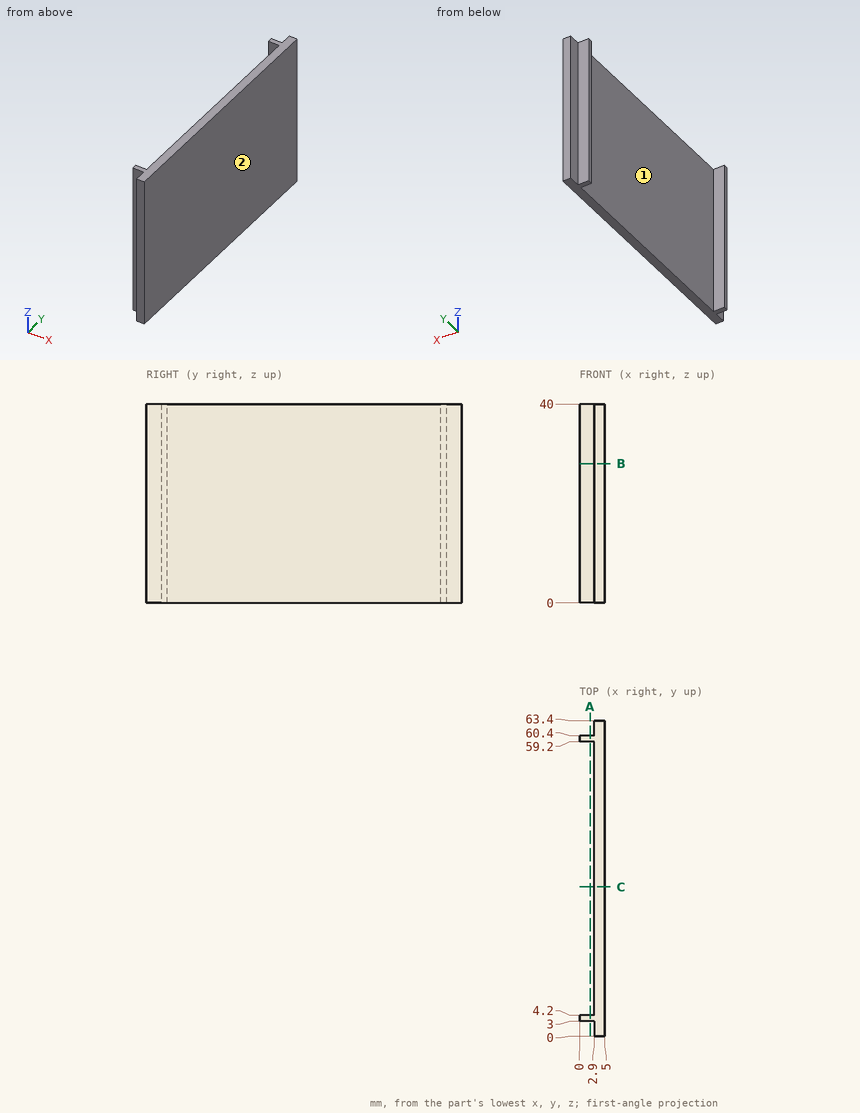
For this review, use the dimensioned drawing (mm, ordinates from the lowest corner) and the shaded views. Coordinates: 2 decimals unless noted, no trailing zeros. Loops run counter-clockwise (first coordinate to the right, second up) from the corner with the lowest first, then second, coordinate; pieces in that order, holes last. Notation, with made-up numbers: (44, 34.5) - (99, 34.5) arc R17 cw to (99, 57.5) - close; hole circle Ø6 at (81.5, 77). An arc over 180 degrees is marked (long way). Use one line per item in the form item = value. Start each with the question number.
1) Draft analysis for pull direction Y (two halves, no side actions). For the marked faces 1 and 2, state which applies: released by +Y, released by -Y, zero draft, split by the parting line, or undercut.
2) For pin 1 (0.9 mm diameter, centred on y = 62, z = 24.5, fed in from -X); pin 2 (3 mm diameter, centred on x = 2, z = 17, fed in from -Y); pin 3 (0.9 mm diameter, centred on x = 1.5, z = 20, fed in from -Y); pin 4 (1.4 mm diameter, centred on x = 2, z = 29, fed in from +Y), all flat-tipped, find the tip position at first contact; note any pin that passes through.
3) To check wall thickness, follow probe 1 along Y at (x, z) = (1.15, 11); probe 2 along X at (y, z) = (59, 29). State the ranges of each line that lie inside material, in increasing order. Write a range as from..to.
4) Take a section at A-A (x = 2.1). State the section outline as (y, z) points, plus the area to 3 significant figures.
5) Take a section at B-B (z = 28). State the section outline as (x, y) points.
6) Take a section at C-C (y = 30). State the section outline as (x, z) points, plus the area to 3 significant figures.
From the geometry:
q1.face_1 = undercut
q1.face_2 = zero draft
q2.pin_1 = 2.9
q2.pin_2 = 0
q2.pin_3 = 3
q2.pin_4 = 60.4
q3.probe_1 = 3..4.2, 59.2..60.4
q3.probe_2 = 2.9..5
q4.outline = (3, 0) - (4.2, 0) - (4.2, 40) - (3, 40) - close; (59.2, 0) - (60.4, 0) - (60.4, 40) - (59.2, 40) - close
q4.area = 96.0 mm2
q5.outline = (0, 3) - (2.9, 3) - (2.9, 0) - (5, 0) - (5, 63.4) - (2.9, 63.4) - (2.9, 60.4) - (0, 60.4) - (0, 59.2) - (2.9, 59.2) - (2.9, 4.2) - (0, 4.2) - close
q6.outline = (2.9, 0) - (5, 0) - (5, 40) - (2.9, 40) - close
q6.area = 84.0 mm2
